from build123d import *

# Parameters (mm, degrees)
F0_R     = 7.5
F0_R_2   = 4
F1_DEPTH = 5
F2_R     = 7
F2_R_2   = 4
F3_DEPTH = 1.1
F4_R     = 7.5
F4_R_2   = 7
F4_R_3   = 4
F5_DEPTH = 32.8
F6_R     = 7
F6_R_2   = 4
F7_DEPTH = 1.1
F8_R     = 7.5
F8_R_2   = 7
F8_R_3   = 4
F9_DEPTH = 5


# Not quite as in the source:
# - a feature names something its author has since deleted; it is built from what else it names


with BuildPart() as f1:
    # F0 (on Front) → F1 (new body)
    with BuildSketch(Plane.XZ):
        Circle(F0_R)
        Circle(F0_R_2, mode=Mode.SUBTRACT)
    extrude(amount=F1_DEPTH)

    # F2 (on face) → F3 (join)
    with BuildSketch(Plane.XZ.offset(5)):
        Circle(F2_R)
        Circle(F2_R_2, mode=Mode.SUBTRACT)
    extrude(amount=F3_DEPTH)

    # F4 (on face) → F5 (join)
    with BuildSketch(Plane.XZ.offset(6.1)):
        Circle(F4_R)
        Circle(F4_R_2, mode=Mode.SUBTRACT)
        Circle(F4_R_2)
        Circle(F4_R_3, mode=Mode.SUBTRACT)
    extrude(amount=F5_DEPTH)

    # F6 (on face) → F7 (join)
    with BuildSketch(Plane.XZ.offset(38.9)):
        Circle(F6_R)
        Circle(F6_R_2, mode=Mode.SUBTRACT)
    extrude(amount=F7_DEPTH)

    # F8 (on face) → F9 (join)
    with BuildSketch(Plane.XZ.offset(40)):
        Circle(F8_R)
        Circle(F8_R_2, mode=Mode.SUBTRACT)
        Circle(F8_R_2)
        Circle(F8_R_3, mode=Mode.SUBTRACT)
    extrude(amount=F9_DEPTH)


solid = f1.part
CAD build for the part. Positions are in the model's coordinates, mm. A direction names the side the tool comes from. Round coordinates to 2 decimals unless told otherwise and drop trailing zeros. Loops run counter-clockwise (first coordinate to the right, second up) from the corner with the lowest first, then second, coordinate; pieces in that order, holes last. Notation, with made-up numbers: (75.5, -8.5) - (123.5, -8.5) arc R22 cw to (123.5, 7.5) - close; hole circle Ø10 at (20, 54). An arc over 180 degrees is marked (long way). Put each result on its own line as item: value.
1. Two-plate mould, pull along Y, no slides. Class faces 1 (the cylindrical face through (-7.493, -42.465, 0.33)), 2 (the flat face through (3, -45, -3)), 3 (the flat face through (7, -38.9, 2)): released by +Y, released by -Y, zero draft, split by the parting line, or undercut.
Geometry check:
face 1: zero draft
face 2: released by -Y
face 3: undercut
2. Slice it at B-B on x = 0. List the corners of the cut face in (y, z).
Geometry check:
outline: (-45, -7.5) - (-40, -7.5) - (-40, -7) - (-38.9, -7) - (-38.9, -7.5) - (-6.1, -7.5) - (-6.1, -7) - (-5, -7) - (-5, -7.5) - (0, -7.5) - (0, -4) - (-45, -4) - close; (-45, 4) - (0, 4) - (0, 7.5) - (-5, 7.5) - (-5, 7) - (-6.1, 7) - (-6.1, 7.5) - (-38.9, 7.5) - (-38.9, 7) - (-40, 7) - (-40, 7.5) - (-45, 7.5) - close
3. Pin check, flat tips, straight feed: P1, Ø1.5, axis at y = -27, z = 3, coming from the +X side; P2, Ø1, axis at x = 2, y = -10, coming from the -Z side; P3, Ø1.5, axis at y = -27.5, z = -1.5, coming from the +X side. Stop position of each tip, or through.
Geometry check:
P1: x = 7.15
P2: z = -7.35
P3: x = 7.46
4. 3-axis set-ups, long thin cutter, end or side, ignore diameter. For faces 4 (the flat face through (7, -40, 2)), 5 (the cylindrical face through (-7.493, -2.465, 0.33)): which of +Z, -Z, +X, -X, +Y, -Y reach the whole face in a straight line?
Geometry check:
face 4: none
face 5: +Y, -Y
5. Wall check: line 1 (Y direction, x = -4.75, z = -5.5); line 2 (Z direction, x = 0, y = -11); line 3 (Z direction, x = 1.5, y = -26.5). Give the ranges that are in metal, low to high.
Geometry check:
line 1: -45 to -40, -38.9 to -6.1, -5 to 0
line 2: -7.5 to -4, 4 to 7.5
line 3: -7.35 to -3.71, 3.71 to 7.35
6. Slice it at D-D on x = -5. List the corners of the cut face in (y, z), and give its area (3 significant figures).
Geometry check:
outline: (-45, -5.59) - (-40, -5.59) - (-40, -4.9) - (-38.9, -4.9) - (-38.9, -5.59) - (-6.1, -5.59) - (-6.1, -4.9) - (-5, -4.9) - (-5, -5.59) - (0, -5.59) - (0, 5.59) - (-5, 5.59) - (-5, 4.9) - (-6.1, 4.9) - (-6.1, 5.59) - (-38.9, 5.59) - (-38.9, 4.9) - (-40, 4.9) - (-40, 5.59) - (-45, 5.59) - close
area: 500 mm²
7. Slice it at A-A on z = 0. List the corners of the cut face in (x, y), and give its area (3 significant figures).
Geometry check:
outline: (-7.5, -45) - (-4, -45) - (-4, 0) - (-7.5, 0) - (-7.5, -5) - (-7, -5) - (-7, -6.1) - (-7.5, -6.1) - (-7.5, -38.9) - (-7, -38.9) - (-7, -40) - (-7.5, -40) - close; (4, -45) - (7.5, -45) - (7.5, -40) - (7, -40) - (7, -38.9) - (7.5, -38.9) - (7.5, -6.1) - (7, -6.1) - (7, -5) - (7.5, -5) - (7.5, 0) - (4, 0) - close
area: 313 mm²
8. Slice it at C-C on y = -32. List the corners of the cut face in (x, z).
Geometry check:
outline: circle Ø15 at (0, 0); hole circle Ø8 at (0, 0)
